from build123d import *

# Parameters (mm, degrees)
SKETCH3_R           = 3
SKETCH3_R_2         = 2.5
BOSS_EXTRUDE2_DEPTH = 3
FILLET1_R           = 10
CUT_EXTRUDE1_DEPTH  = 10
FILLET2_R           = 3.75


with BuildPart() as part:
    # Sketch3 → Boss-Extrude2 (new body)
    with BuildSketch(Plane(origin=(0, 0, 0), x_dir=(0, 0, -1), z_dir=(1, 0, 0))):
        with BuildLine():
            Line((7.171582169, 19.591665787), (82.171582169, 41.707880218))
            ThreePointArc((82.171582169, 41.707880218), (85.373366716, 42.109241865), (88.536274395, 41.470077986))
            Line((88.536274395, 41.470077986), (147.036274395, 19.353863555))
            ThreePointArc((147.036274395, 19.353863555), (152.853863555, 6.463725605), (139.963725605, 0.646136445))
            Line((139.963725605, 0.646136445), (100.980229255, 15.384040113))
            Line((100.980229255, 15.384040113), (100.980229255, -1.493532665))
            ThreePointArc((100.980229255, -1.493532665), (90.980229255, -11.493532665), (80.980229255, -1.493532665))
            Line((80.980229255, -1.493532665), (80.980229255, 20.505135217))
            Line((80.980229255, 20.505135217), (12.828417831, 0.408334213))
            ThreePointArc((12.828417831, 0.408334213), (0.408334213, 7.171582169), (7.171582169, 19.591665787))
        make_face()
        with Locations((85, 32.116214431)):
            Circle(SKETCH3_R, mode=Mode.SUBTRACT)
        with Locations((90.980229255, -1.493532665)):
            Circle(SKETCH3_R_2, mode=Mode.SUBTRACT)
        with Locations((10, 10)):
            Circle(SKETCH3_R_2, mode=Mode.SUBTRACT)
        with Locations((143.5, 10)):
            Circle(SKETCH3_R_2, mode=Mode.SUBTRACT)
    extrude(amount=BOSS_EXTRUDE2_DEPTH)

    # Fillet1
    fillet1_edges = [part.edges().sort_by_distance(p)[0] for p in [
        (1.5, 20.505135217, -80.980229255),
        (1.5, 15.384040113, -100.980229255),
    ]]
    fillet(fillet1_edges, radius=FILLET1_R)

    # Sketch5 → Cut-Extrude1 (cut)
    with BuildSketch(Plane(origin=(0, 0, 0), x_dir=(0, 0, -1), z_dir=(1, 0, 0))):
        Polygon((23.326841994, 17.839501416), (61.693505144, 29.153172739), (63.814818517, 21.959423399), (25.448155367, 10.645752076), align=None)
        with BuildLine():
            Line((86.060882319, 34.922373497), (109.445541205, 26.081687509))
            Line((109.445541205, 26.081687509), (90.980229255, 11.910433147))
            Line((90.980229255, 11.910433147), (82.273860108, 30.863951963))
            ThreePointArc((82.273860108, 30.863951963), (82.806608326, 34.162927153), (86.060882319, 34.922373497))
        make_face()
    extrude(amount=CUT_EXTRUDE1_DEPTH, mode=Mode.SUBTRACT)

    # Fillet2
    fillet2_edges = [part.edges().sort_by_distance(p)[0] for p in [
        (1.5, 11.910433147, -90.980229255),
        (1.5, 26.081687509, -109.445541205),
        (1.5, 29.153172739, -61.693505144),
        (1.5, 21.959423399, -63.814818517),
        (1.5, 10.645752076, -25.448155367),
        (1.5, 17.839501416, -23.326841994),
    ]]
    fillet(fillet2_edges, radius=FILLET2_R - 0.0001)  # a hair under: the kernel refuses the full size


solid = part.part
The listing builds one solid part. Answer for the finished solid, in the listing's coordinates (mm). A direction names the side the tool comes from. Coordinates: 2 decimals unless noted, no trailing zeros. Write each loop counter-clockwise with the first axis right and the second up, starting at its lowest first coordinate (ties: lowest second). Pieces come first, ordered by that corner, then holes. Notation, with made-up numbers: M -37.75,-30 L -25.75,-30 A13 cw -25.75,-12 Z; hole C 79.25,18 d9. An arc over 180 degrees is marked long. Write each question's results on one line, items separated by ' | '.
Item 1: The part is cut by section B-B on z = -10. Determine the outline of the cut face in (x, y), and give its area (3 significant figures).
Answer below:
outline: M 0,0 L 3,0 L 3,7.5 L 0,7.5 Z; M 0,12.5 L 3,12.5 L 3,20.43 L 0,20.43 Z | area: 46.3 mm2
Item 2: Consider probe 1 along Y at (x, z) = (1.6, -10); probe 2 along Y at (x, z) = (2.25, -143.5); probe 3 along Z at (x, y) = (2.3, -6). Determine where each line is inside the solid, lowest interval first. Write a range as [from, to].
Answer below:
probe 1: [0, 7.5], [12.5, 20.43] | probe 2: [0, 7.5], [12.5, 20.69] | probe 3: [-99.91, -82.05]
Item 3: For a pull along Y with two mould halves and no side action, classify faces 1 (the face through (1.48, 31.74, -94.48)), 2 (the face through (1.479, 30.495, -44.147)), 3 (the face through (1.48, 5.39, -127.42)) as released by +Y, released by -Y, zero draft, split by the parting line, or undercut.
Answer below:
face 1: undercut | face 2: released by +Y | face 3: released by -Y
Item 4: The part is cut by section A-A on x = 0.6. State how many separate pieces and enclosed holes the cut face has, and give its area (3 significant figures).
Answer below:
separate pieces: 1 | enclosed holes: 5 | area: 3,140 mm2
Item 5: Given P1, Ø1, axis at x = 1, y = 17.5, coming from the -Z side; P2, Ø0.9, axis at x = 2, y = 1.5, coming from the +Z side; P3, Ø0.7, axis at x = 1.5, y = -0.5, coming from the -Z side; P4, Ø8, axis at y = -1.49, z = -90.98, coming from the -X side, each flat-ended and moving along its own axis, determine where each tip first touches the part or whether it passes through.
Answer below:
P1: z = -150.64 | P2: z = -4.07 | P3: z = -100.98 | P4: x = 0
Item 6: The part is cut by section D-D on z = -126.5. Determine the outline of the cut face in (x, y), and give its area (3 significant figures).
Answer below:
outline: M 0,5.74 L 3,5.74 L 3,27.12 L 0,27.12 Z | area: 64.1 mm2
Item 7: Which of the six approach directions +Z, -Z, +X, -X, +Y, -Y give full straight-line access (tool end or side, diameter ignored) to faces 4 (the face through (1.479, 16.367, -44.85)), 5 (the face through (1.48, -11.49, -91.2))?
Answer below:
face 4: +X, -X | face 5: +X, -X, -Y
Item 8: The part is cut by section C-C on z = -30.5. Determine the outline of the cut face in (x, y).
Answer below:
outline: M 0,5.62 L 3,5.62 L 3,12.14 L 0,12.14 Z; M 0,19.95 L 3,19.95 L 3,26.47 L 0,26.47 Z
